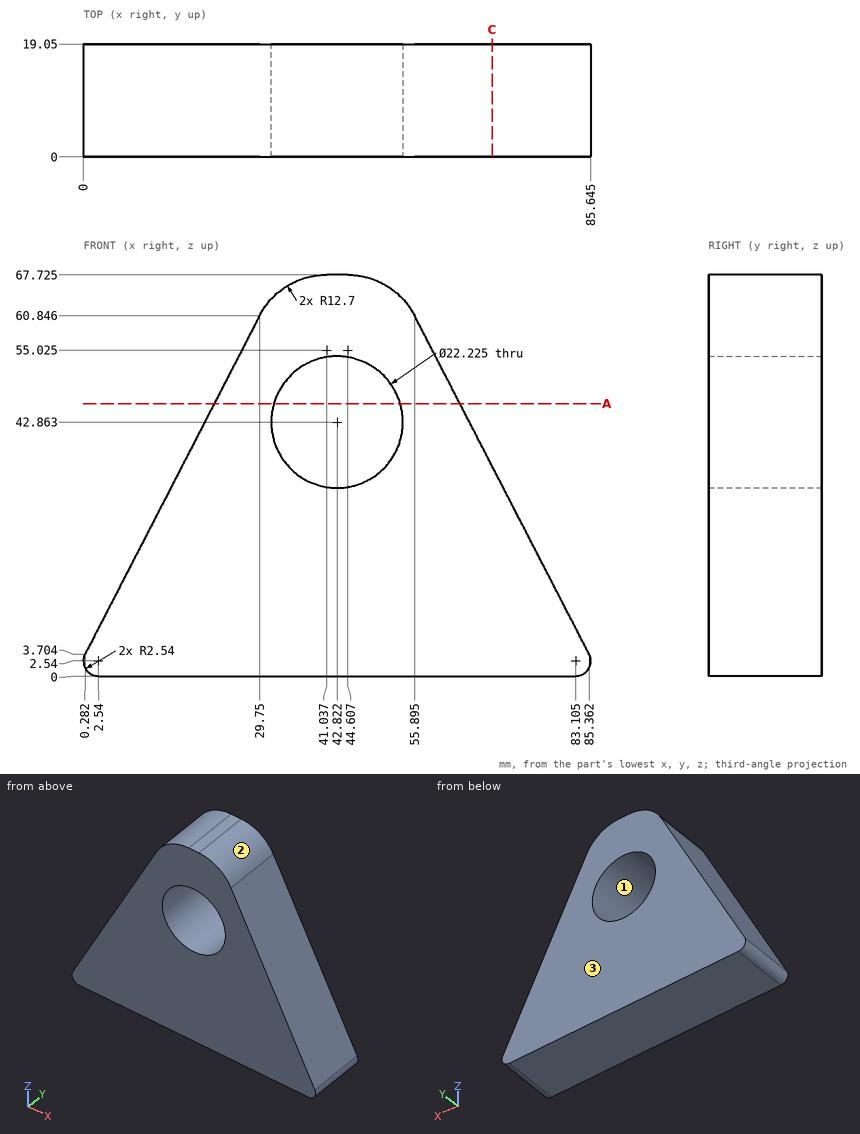
Print and shaded views of the part. All mm, measured from the part's lowest x, y and z. Give positions to 0.01 mm unless a question says otherwise; leave off trailing zeros. Write each loop counter-clockwise with the first axis right and the second up, starting at its lowest first coordinate (ties: lowest second). Pieces come first, ordered by that corner, then holes. Notation, with made-up numbers: (34.25, -4) -> (92.25, -4) arc R26 cw to (92.25, 33) -> close; hole circle Ø9 at (-6, 20). An arc over 180 degrees is marked (long way). Write item = value, one per line.
(1) Probe line 1 along X through (y, z) = (18, 43.5) (1 decimal); line 2 along X through (y, z) = (7.5, 34.5) (1 decimal); line 3 along Z through (x, y) = (48, 6.25) (1 decimal). List the from-to ranges inside material, lowest first.
Determined:
line_1 = 20.8 to 31.7, 53.9 to 64.8
line_2 = 16.2 to 35.5, 50.1 to 69.5
line_3 = 0 to 33, 52.7 to 67.3
(2) Mould opens along Z. For the marked faces 1, 2 and 3 say: released by +Z, released by -Z, zero draft, split by the parting line, or undercut.
Determined:
face_1 = undercut
face_2 = released by +Z
face_3 = zero draft
(3) Slice it at A-A, the plane z = 46. Give the cut face in (x, y).
Determined:
outline = (22.09, 0) -> (32.16, 0) -> (32.16, 19.05) -> (22.09, 19.05) -> close; (53.48, 0) -> (63.55, 0) -> (63.55, 19.05) -> (53.48, 19.05) -> close
(4) Slice it at C-C, the plane x = 69. Give the cut face in (y, z).
Determined:
outline = (0, 0) -> (19.05, 0) -> (19.05, 35.43) -> (0, 35.43) -> close
(5) Flat gauge pins, fed straight in: P1, Ø2, axis at y = 11, z = 55, coming from the +X side (1 decimal); P2, Ø1, axis at y = 2, z = 57.5, coming from the +X side; P3, Ø4, axis at y = 3, z = 32.5, coming from the +X side (1 decimal). Where does each tip first touch, or does it go through?
Determined:
P1 = 59.4
P2 = 57.88
P3 = 71.5
